Source: three-view drawing plus pictorial views. Frame: mm from the lowest corner of the part. Give positions to 0.01 mm unless a question says otherwise; leave off trailing zeros. Order: outer loops, then holes, each group sorted by start corner. A loop starts at its lowest first (then second) coordinate and runs counter-clockwise, first axis right, second up. Notation, with made-up numbers: (53.5, 44.25) - (78.5, 44.25) arc R19 cw to (78.5, 54.25) - close; hole circle Ø7 at (70.5, -1). An arc over 180 degrees is marked (long way). Use CSV: the item, a comma, the result in double quotes.
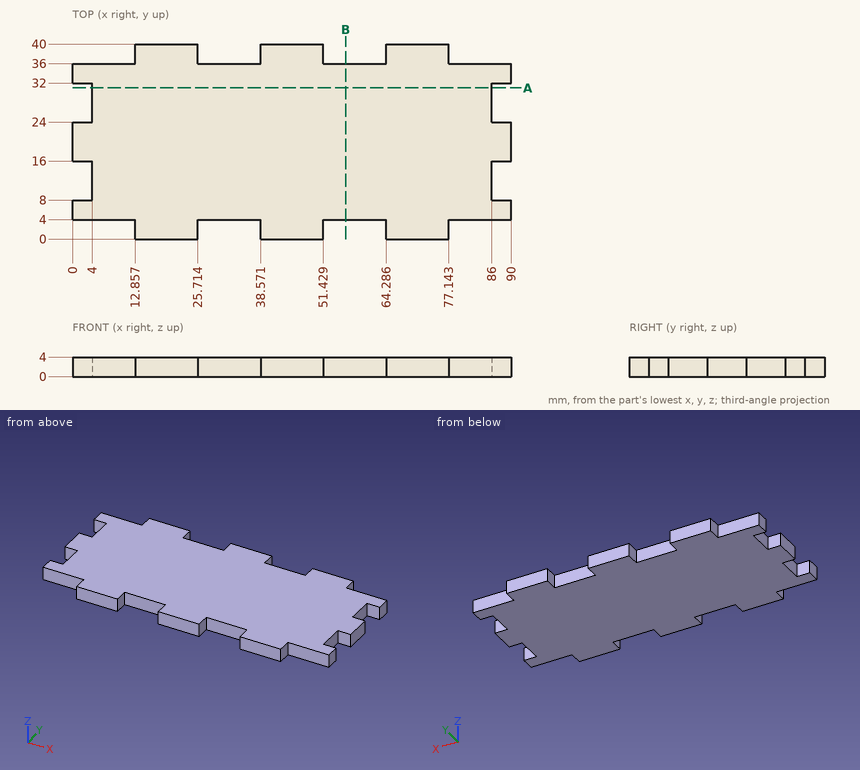
Item 1: Section B-B on x = 56. Return the cut outline in (y, z), then the cut area to 3 significant figures.
Filled in:
outline,"(4, 0) - (36, 0) - (36, 4) - (4, 4) - close"
area,"128 mm2"
Item 2: First-contact query: pin 1 (1.2 mm diameter, centred on y = 37.5, z = 2.5, fed in from -X); pin 2 (2 mm diameter, centred on x = 31.5, z = 2, fed in from +Y); pin 3 (1.2 mm diameter, centred on y = 2.5, z = 1.5, fed in from +X); pin 4 (8 mm diameter, centred on x = 44, y = 14.5, fed in from -Z). Flat tips, straight axial feed; report the tip coordinate or a pass-through.
Filled in:
pin 1,"stops at x = 12.86"
pin 2,"stops at y = 36"
pin 3,"stops at x = 77.14"
pin 4,"stops at z = 0"
Item 3: Section A-A on y = 31. Return the cut outline in (x, z), then the cut area to 3 significant figures.
Filled in:
outline,"(4, 0) - (86, 0) - (86, 4) - (4, 4) - close"
area,"328 mm2"
Item 4: Material intervals for line 1 (X direction, y = 3, z = 0.65) (1 decimal); line 2 (X direction, y = 12, z = 2.6); line 3 (Y direction, x = 81.5, z = 1.95), sorted ascending. Write a range as from..to.
Filled in:
line 1,"x = 12.9..25.7, 38.6..51.4, 64.3..77.1"
line 2,"x = 4..86"
line 3,"y = 4..36"
